Check sheet for the drawn part. Datum: minimum x, y, z corner. Units: mm. Give positions to 0.01 mm unless a question says otherwise; leave off trailing zeros. Loops run counter-clockwise (first coordinate to the right, second up) from the corner with the lowest first, then second, coordinate; pieces in that order, holes last. Notation, with made-up numbers: (61.5, -2.5) - (65.5, -2.5) arc R15 ccw to (65.5, 25.5) - close; hole circle Ø2 at (1.25, -36.5). An arc over 180 degrees is marked (long way). One line per item, written item: value. Start each with the question number.
1. Sectioned sample at C-C (z = 17). Record the cut outline in (x, y).
2. Sectioned sample at B-B (y = 4.1). Count the separate pieces of the cut face and the enclosed holes in it, plus the area to 3 significant figures.
3. Sectioned sample at A-A (x = 44.45). Record the cut outline in (y, z).
4. Gauge pin test, flat ends, axial feed: pin 1 (3 mm diameter, centred on x = 44.45, z = 59.76, fed in from -Y); pin 2 (3.5 mm diameter, centred on x = 56.83, z = 17.27, fed in from +Y); pin 3 (3 mm diameter, centred on x = 2.5, y = 4, fed in from +Z); pin 4 (3 mm diameter, centred on y = 2, z = 59, fed in from +X). Record the tip position at first contact, or that the pin passes through.
5. Sectioned sample at D-D (x = 29). Record the cut outline in (y, z), plus the area to 3 significant figures.
6. Scan lines: L1, parallel to Z at x = 44.5, y = 5.05 (1 decimal); L2, parallel to Z at x = 45.5, y = 4.9 (1 decimal); L3, parallel to X at y = 1, z = 12. Record each from-to range of solid material in increasing order. Write a range as [from, to].
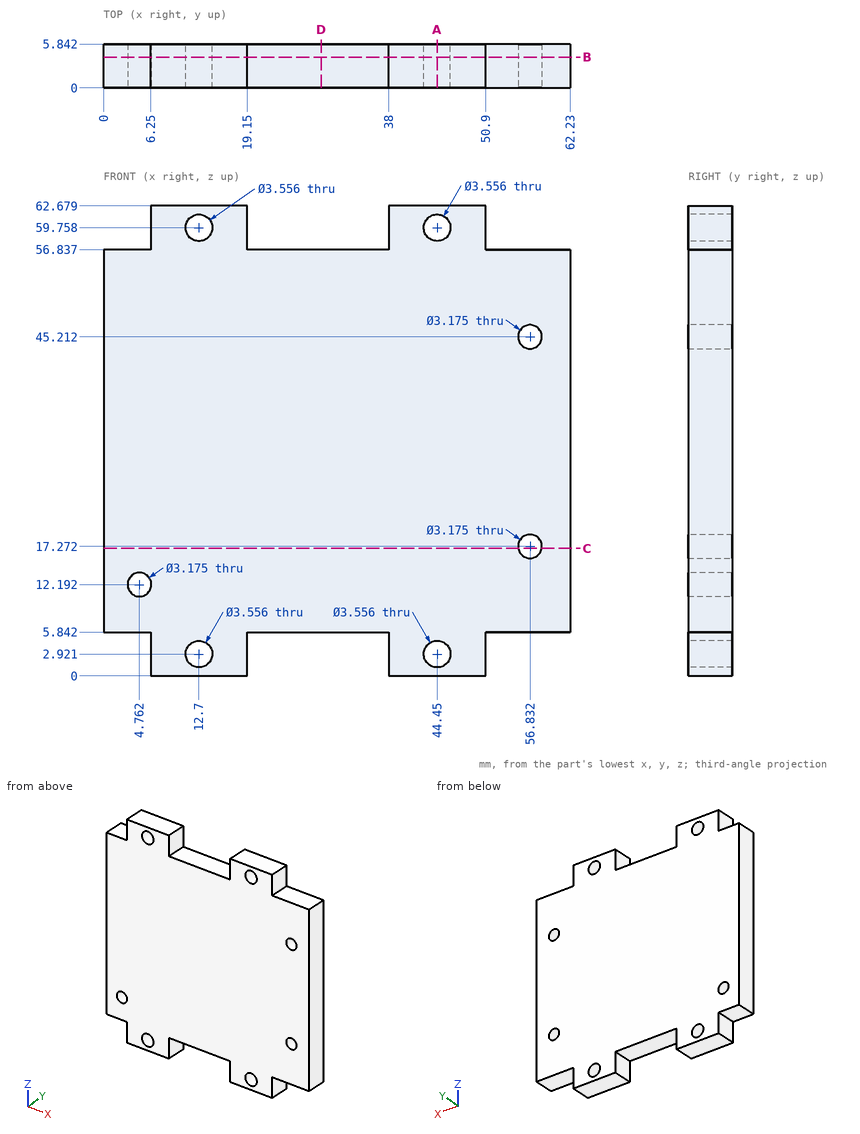
Results are:
1. outline: (0, 0) - (55.27, 0) - (55.27, 5.84) - (0, 5.84) - close; (58.4, 0) - (62.23, 0) - (62.23, 5.84) - (58.4, 5.84) - close
2. separate pieces: 1
2. enclosed holes: 7
2. area: 3,410 mm^2
3. outline: (0, 0) - (5.84, 0) - (5.84, 1.14) - (0, 1.14) - close; (0, 4.7) - (5.84, 4.7) - (5.84, 57.98) - (0, 57.98) - close; (0, 61.54) - (5.84, 61.54) - (5.84, 62.68) - (0, 62.68) - close
4. pin 1: passes through
4. pin 2: stops at y = 5.84
4. pin 3: stops at z = 56.84
4. pin 4: stops at x = 50.9
5. outline: (0, 5.84) - (5.84, 5.84) - (5.84, 56.84) - (0, 56.84) - close
5. area: 298 mm^2
6. L1: z = [0, 1.1], [4.7, 58], [61.5, 62.7]
6. L2: z = [0, 1.5], [4.4, 58.3], [61.2, 62.7]
6. L3: x = [0, 3.19], [6.34, 62.23]
